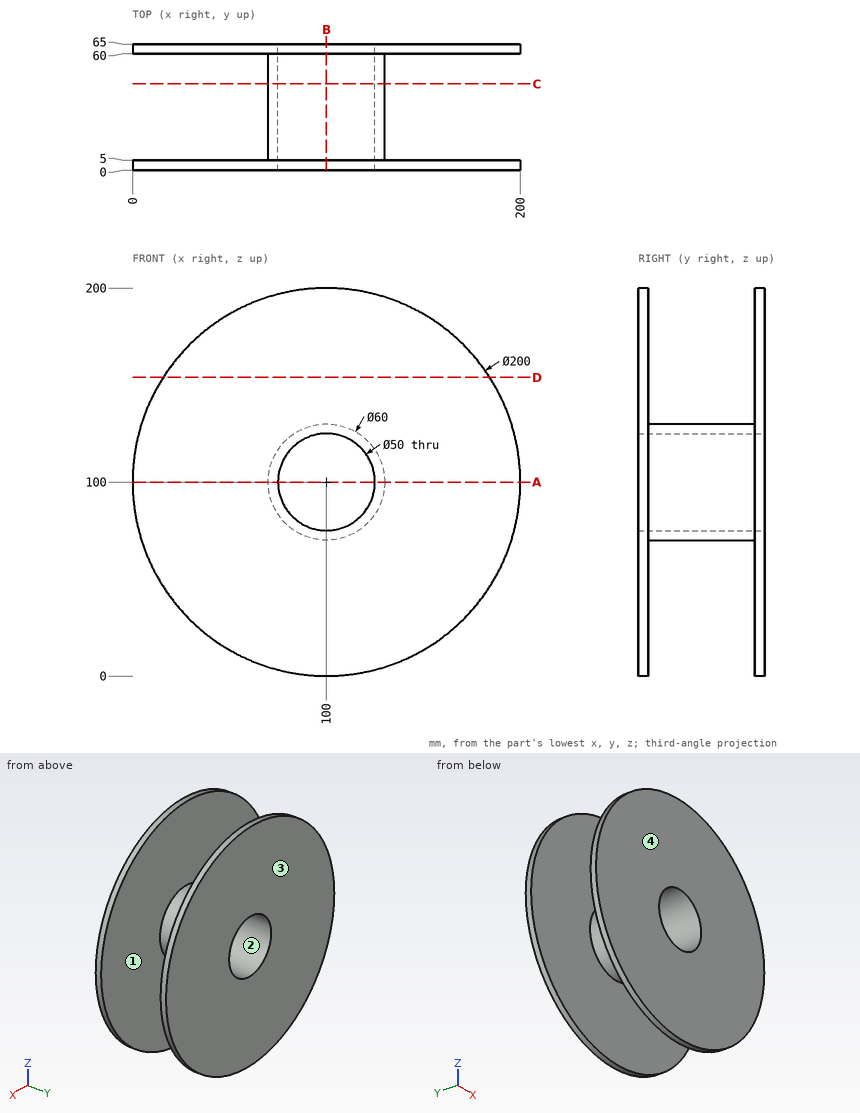
Design review of the part shown in the three views and the two pictorial views. Dimensions are in mm from the part's minimum x, y and z. Round coordinates to 2 decimals unless told otherwise and drop trailing zeros. Order: outer loops, then holes, each group sorted by start corner. A loop starts at its lowest first (then second) coordinate and runs counter-clockwise, first axis right, second up. Notation, with made-up numbers: (74, 34) -> (126, 34) arc R9 ccw to (126, 42) -> close; hole circle Ø5 at (65.25, 54). An arc over 180 degrees is marked (long way). Write item = value, one per line. Start each with the question number.
1) To check wall thickness, follow line 1 (Y direction, x = 129.5, z = 158); line 2 (Z direction, x = 100, y = 20); line 3 (Z direction, x = 85, y = 53). State the ranges of each line that lie inside material, in increasing order. Write a range as from..to.
2) The part is to be moulded in two halves that separate along Y. For the marked faces 1, 2, 3 and 4, say which applies: +Y half, -Y half, draft (parallel to the pull), parting line (faces both ways), or undercut.
3) Take a section at C-C on y = 44.5. State the section outline as (x, z) points.
4) Insertion check: pin 1 (10 mm diameter, centred on x = 72.5, y = 7, fed in from +Z); pin 2 (12 mm diameter, centred on y = 53, z = 66.5, fed in from +X); pin 3 (8 mm diameter, centred on x = 122, y = 22.5, fed in from -Z). Each pin has a flat end and moves straight along its axis. Give the tip position at first contact, or say it passes through.
5) Take a section at A-A on z = 100. State the section outline as (x, y) points.
6) Take a section at B-B on x = 100. State the section outline as (y, z) points.
7) Take a section at D-D on z = 154. State the section outline as (x, y) points, plus the area to 3 significant figures.
Verdict:
q1.line_1 = 0..5, 60..65
q1.line_2 = 70..75, 125..130
q1.line_3 = 74.02..80, 120..125.98
q2.face_1 = undercut
q2.face_2 = draft
q2.face_3 = +Y half
q2.face_4 = -Y half
q3.outline = circle Ø60 at (100, 100); hole circle Ø50 at (100, 100)
q4.pin_1 = 197.34
q4.pin_2 = 111.99
q4.pin_3 = 76
q5.outline = (0, 0) -> (75, 0) -> (75, 65) -> (0, 65) -> (0, 60) -> (70, 60) -> (70, 5) -> (0, 5) -> close; (125, 0) -> (200, 0) -> (200, 5) -> (130, 5) -> (130, 60) -> (200, 60) -> (200, 65) -> (125, 65) -> close
q6.outline = (0, 0) -> (5, 0) -> (5, 70) -> (60, 70) -> (60, 0) -> (65, 0) -> (65, 75) -> (0, 75) -> close; (0, 125) -> (65, 125) -> (65, 200) -> (60, 200) -> (60, 130) -> (5, 130) -> (5, 200) -> (0, 200) -> close
q7.outline = (15.83, 0) -> (184.17, 0) -> (184.17, 5) -> (15.83, 5) -> close; (15.83, 60) -> (184.17, 60) -> (184.17, 65) -> (15.83, 65) -> close
q7.area = 1,680 mm2
